Autodesk Inventor part; units mm, degrees
ref_plane "YZ Plane" through (0, 0, 0) normal (1, 0, 0) x (0, 1, 0)
ref_plane "XZ Plane" through (0, 0, 0) normal (0, 1, 0) x (-1, 0, 0)
ref_plane "XY Plane" through (0, 0, 0) normal (0, 0, 1) x (1, 0, 0)
ref_plane "Work Plane1" through (-527.421, 38.0398, -128.7467) normal (0, 0, 1) x (0.9994, -0.0351, 0)
sketch "Sketch1" plane through (-527.421, 38.0398, -128.7467) normal (0, 0, 1) x (0.9994, -0.0351, 0)
  line L0 (-71.9298, -7.1441) -> (116.8182, 283.622)
  line L1 (116.8182, 283.622) -> (240.6596, 287.9699)
  line L2 (449.4274, 297.701) -> (252.1683, 290.7755)
  line L3 (607.7587, -12.8972) -> (449.4274, 297.701)
  line L4 (625.2338, -510.6359) -> (607.7587, -12.8972)
  line L5 (-56.2402, -454.0286) -> (-71.9298, -7.1441)
  point P0 (528.431, -19.5106)
sketch "Sketch2" plane through (-527.421, 38.0398, -128.7467) normal (0, 0, 1) x (0.9994, -0.0351, 0)
  line L0 (-71.9298, -7.1441) -> (116.8182, 283.622)
  line L1 (-56.2402, -454.0286) -> (-71.9298, -7.1441)
  line L2 (116.8182, 283.622) -> (240.6596, 287.9699)
  line L3 (607.7587, -12.8972) -> (449.4274, 297.701)
  line L4 (625.2338, -510.6359) -> (607.7587, -12.8972)
  line L5 (625.2338, -510.6359) -> (-56.2402, -534.5617)
  line L6 (-56.2402, -534.5617) -> (-56.2402, -454.0286)
  line L7 (116.8182, 283.622) -> (449.4274, 297.701)
  point P0 (528.431, -19.5106)
extrude "Extrusion1" add sketch "Sketch2" against normal blind 1.6
properties part number "cover end plates-02"
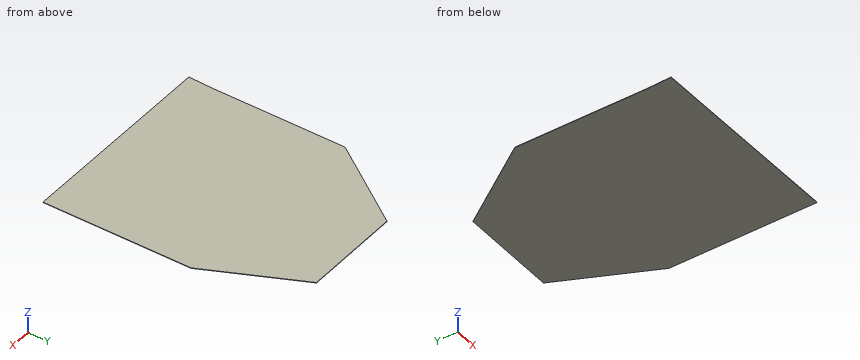
Build history of the part. All positions in model axes, mm. Round coordinates to 2 decimals unless told otherwise and drop trailing zeros. Loops run counter-clockwise (first coordinate to the right, second up) from the corner with the lowest first, then second, coordinate; pieces in that order, holes last.
Item 1: Saw through at A-A (z = -129.6). List the corners of the cut face in (x, y), then the cut area to 3 significant figures.
Item 2: Pin check, flat tip, straight feed: P1, Ø0.5, axis at y = -294.5, z = -129, coming from the +X side. Stop position of the tip, or through.
Item 3: Saw through at B-B (y = 190.5). List the corners of the cut face in (x, z).
Item 4: Saw through at C-C (x = -541.5). List the corners of the cut face in (y, z), then the cut area to 3 significant figures.
Item 5: Drill centre lines: line 1 along X through (y, z) = (-98, -129.5); line 2 along Y through (x, z) = (-209, -128.8); line 3 along X through (y, z) = (153, -129.55). Where is each one in solid material? Low to high.
Worked answers:
1. outline: (-602.39, -494.22) - (79.5, -494.23) - (79.51, 3.82) - (-67.82, 319.78) - (-400.72, 317.39) - (-599.56, 33.42) - (-599.56, -413.74) - close
1. area: 500,000 mm2
2. P1: stops at x = 79.51
3. outline: (-489.57, -130.35) - (-7.54, -130.35) - (-7.54, -128.75) - (-489.57, -128.75) - close
4. outline: (-494.22, -130.35) - (116.34, -130.35) - (116.34, -128.75) - (-494.22, -128.75) - close
4. area: 977 mm2
5. line 1: x = -599.56 to 79.51
5. line 2: y = -494.22 to 318.77
5. line 3: x = -515.83 to 9.95
